Geometry check sheet. Reference: the model listing, model coordinates, mm. Face numbers are marked on the shaded views. Coordinates: 2 decimals unless noted, no trailing zeros. Write each loop counter-clockwise with the first axis right and the second up, starting at its lowest first coordinate (ties: lowest second). Pieces come first, ordered by that corner, then holes.
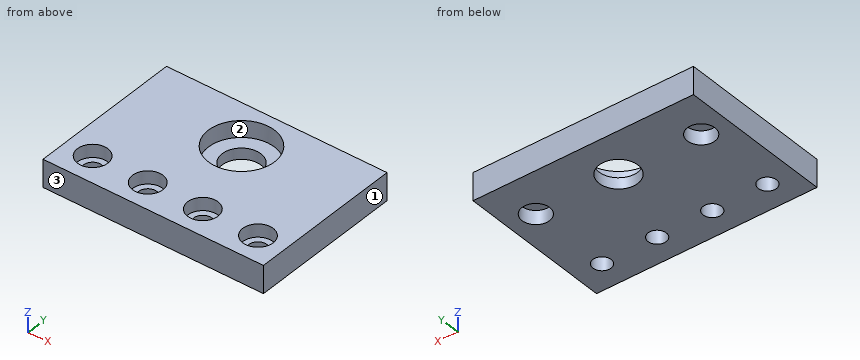
from build123d import *

# Parameters (mm, degrees)
SKETCH_1_W                   = 80
SKETCH_1_H                   = 56
EXTRUDE_1_DEPTH              = 10
HOLE_WIZARD_M6_1_D           = 6.6
HOLE_WIZARD_M6_1_CBORE_D     = 11
HOLE_WIZARD_M6_1_CBORE_DEPTH = 4.7
SKETCH_5_R                   = 7
CUT_EXTRUDE_1_DEPTH          = 10
SKETCH_6_R                   = 12
CUT_EXTRUDE_2_DEPTH          = 6
SKETCH_7_R                   = 5
CUT_EXTRUDE_3_DEPTH          = 5


with BuildPart() as part:
    # 草图1 → 凸台-拉伸1 (new body)
    with BuildSketch(Plane.XY):
        with Locations((0, -12)):
            Rectangle(SKETCH_1_W, SKETCH_1_H)
    extrude(amount=-EXTRUDE_1_DEPTH)

    # M6 内六角花型圆柱头螺钉的柱形沉头孔1 (through all)
    with Locations(Plane.XY):
        with Locations((30, -30), (-30, -30), (10, -30), (-10, -30)):
            CounterBoreHole(HOLE_WIZARD_M6_1_D / 2, HOLE_WIZARD_M6_1_CBORE_D / 2, HOLE_WIZARD_M6_1_CBORE_DEPTH)

    # 草图5 → 切除-拉伸1 (cut)
    with BuildSketch(Plane.XY):
        Circle(SKETCH_5_R)
    extrude(amount=-CUT_EXTRUDE_1_DEPTH, mode=Mode.SUBTRACT)

    # 草图6 → 切除-拉伸2 (cut)
    with BuildSketch(Plane(origin=(0, 0, 0), x_dir=(-1, 0, 0), z_dir=(0, 0, -1))):
        Circle(SKETCH_6_R)
    extrude(amount=CUT_EXTRUDE_2_DEPTH, mode=Mode.SUBTRACT)

    # 草图7 → 切除-拉伸3 (cut)
    with BuildSketch(Plane(origin=(0, 0, -10), x_dir=(-1, 0, 0), z_dir=(0, 0, -1))):
        with Locations((30, 0)):
            Circle(SKETCH_7_R)
    cut_extrude_3 = extrude(amount=-CUT_EXTRUDE_3_DEPTH, mode=Mode.SUBTRACT)

    # 镜向1: 切除-拉伸3 across plane
    add(cut_extrude_3.mirror(Plane(origin=(0, 0, 0), x_dir=(0, 0, 1), z_dir=(1, 0, 0))), mode=Mode.SUBTRACT)


solid = part.part
1. Draft check along X on the marked faces 1, 2 and 3. Enter one of: released by +X, released by -X, zero draft, split by the parting line, or undercut.
Computed values:
face 1: released by +X
face 2: undercut
face 3: zero draft
2. Gauge pin test, flat ends, axial feed: pin 1 Ø10 at (x, y) = (-11.5, -7) entering from +Z; pin 2 Ø9 at (x, y) = (-10, -30) entering from +Z; pin 3 Ø3 at (x, y) = (32, -2.5) entering from -Z; pin 4 Ø21.5 at (x, y) = (0, 0) entering from +Z. Record the tip position at first contact, or that the pin passes through.
Computed values:
pin 1: stops at z = 0
pin 2: stops at z = -4.7
pin 3: stops at z = -5
pin 4: stops at z = -6
3. Sectioned sample at A-A, the plane y = 0. Record the boundary of the cut face in (x, z).
Computed values:
outline: (-40, -10) - (-35, -10) - (-35, -5) - (-25, -5) - (-25, -10) - (-7, -10) - (-7, -6) - (-12, -6) - (-12, 0) - (-40, 0) - close; (7, -10) - (25, -10) - (25, -5) - (35, -5) - (35, -10) - (40, -10) - (40, 0) - (12, 0) - (12, -6) - (7, -6) - close
4. Sectioned sample at D-D, the plane x = -10.5. Record the boundary of the cut face in (y, z).
Computed values:
outline: (-40, -10) - (-33.26, -10) - (-33.26, -4.7) - (-35.48, -4.7) - (-35.48, 0) - (-40, 0) - close; (-26.74, -10) - (16, -10) - (16, 0) - (5.81, 0) - (5.81, -6) - (-5.81, -6) - (-5.81, 0) - (-24.52, 0) - (-24.52, -4.7) - (-26.74, -4.7) - close
5. Sectioned sample at B-B, the plane x = 30. Record the boundary of the cut face in (y, z).
Computed values:
outline: (-40, -10) - (-33.3, -10) - (-33.3, -4.7) - (-35.5, -4.7) - (-35.5, 0) - (-40, 0) - close; (-26.7, -10) - (-5, -10) - (-5, -5) - (5, -5) - (5, -10) - (16, -10) - (16, 0) - (-24.5, 0) - (-24.5, -4.7) - (-26.7, -4.7) - close
6. Sectioned sample at C-C, the plane z = -9. Record the boundary of the cut face in (x, y).
Computed values:
outline: (-40, -40) - (40, -40) - (40, 16) - (-40, 16) - close; hole circle Ø10 at (-30, 0); hole circle Ø6.6 at (-30, -30); hole circle Ø6.6 at (-10, -30); hole circle Ø14 at (0, 0); hole circle Ø6.6 at (10, -30); hole circle Ø10 at (30, 0); hole circle Ø6.6 at (30, -30)
7. Thickness scan on line 1 along Y through (x, z) = (-30, -8.7); line 2 along X through (y, z) = (-0.5, -5.5); line 3 along Y through (x, z) = (0, -8.25). Record the ranges inside material, lowest first.
Computed values:
line 1: y = -40 to -33.3, -26.7 to -5, 5 to 16
line 2: x = -40 to -34.97, -25.03 to -11.99, 11.99 to 25.03, 34.97 to 40
line 3: y = -40 to -7, 7 to 16
